Design review of the part built by this model. Coordinates are the model's own, in mm. Face numbers are marked on the shaded views. A direction names the side the tool comes from. Give positions to 0.01 mm unless a question says otherwise; leave off trailing zeros. Loops run counter-clockwise (first coordinate to the right, second up) from the corner with the lowest first, then second, coordinate; pieces in that order, holes last. Notation, with made-up numbers: (69, 37) -> (93, 37) arc R35 ccw to (93, 74) -> close; hole circle Ø11 at (-14.75, -34.5). An arc over 180 degrees is marked (long way). Use a Markdown table: item, result. Add a question column.
1. For pin 1 Ø4 at (x, y) = (-48.5, 7.5) entering from +Z; pin 2 Ø3.5 at (y, z) = (3, -6.5) entering from -X; pin 3 Ø3.5 at (x, y) = (46, -7.5) entering from +Z; pin 4 Ø3 at (x, y) = (5, 9.5) entering from -Z, all flat-tipped, find the tip position at first contact; note any pin that passes through.
2. Add section A-A (z = -4.5). State the section outline as (x, y) points.
3. Add section D-D (x = 48.5). State the section outline as (y, z) points.
4. Draft analysis for pull direction X (two halves, no side actions). For the marked faces 4, 5, 6 and 7, state which applies: pulls with the +X half, pulls with the -X half, needs draft (parallel to the pull), parting line crosses it, or undercut.
5. Add section C-C (z = -11.25). State the section outline as (x, y) points.
6. Add section B-B (x = 0). State the section outline as (y, z) points, and give its area (3 significant figures).
7. To check wall thickness, follow line 1 (Y direction, x = -48.5, z = -10.05); line 2 (X direction, y = 4, z = -4); line 3 (Y direction, x = 5.5, z = 2.8). State the ranges of each line that lie inside material, in increasing order.
8. For the marked faces 1, 2 and 3, list the 3-axis set-ups (+Z, -Z, +X, -X, +Y, -Y) from which the entire face can be reached by the end or side of a thin tool; tool diameter is ignored.
```python
from build123d import *

# Parameters (mm, degrees)
SKETCH1_W           = 85
SKETCH1_H           = 30
SKETCH1_R           = 6
BOSS_EXTRUDE1_DEPTH = 3.2
SKETCH5_R           = 1.75
CUT_EXTRUDE1_DEPTH  = 4.2
SKETCH7_R           = 3
CUT_EXTRUDE2_DEPTH  = 2
SKETCH2_W           = 4
SKETCH2_H           = 30
BOSS_EXTRUDE2_DEPTH = 12.3
SKETCH3_W           = 16
SKETCH3_H           = 30
SKETCH3_R           = 2.25
BOSS_EXTRUDE3_DEPTH = 4
CHAMFER1_SIZE       = 5


with BuildPart() as part:
    # Sketch1 → Boss-Extrude1 (new body)
    with BuildSketch(Plane.XY):
        Rectangle(SKETCH1_W, SKETCH1_H)
        Circle(SKETCH1_R, mode=Mode.SUBTRACT)
    extrude(amount=BOSS_EXTRUDE1_DEPTH)

    # Sketch5 → Cut-Extrude1 (cut, through all)
    with BuildSketch(Plane.XY.offset(3.2)):
        with Locations((5.5, 9.526279442)):
            Circle(SKETCH5_R)
        with Locations((-11, 0)):
            Circle(SKETCH5_R)
        with Locations((5.5, -9.526279442)):
            Circle(SKETCH5_R)
    extrude(amount=-CUT_EXTRUDE1_DEPTH, mode=Mode.SUBTRACT)

    # Sketch7 → Cut-Extrude2 (cut)
    with BuildSketch(Plane(origin=(0, 0, 0), x_dir=(-1, 0, 0), z_dir=(0, 0, -1))):
        with Locations((-5.5, 9.526279442)):
            Circle(SKETCH7_R)
        with Locations((11, 0)):
            Circle(SKETCH7_R)
        with Locations((-5.5, -9.526279442)):
            Circle(SKETCH7_R)
    extrude(amount=-CUT_EXTRUDE2_DEPTH, mode=Mode.SUBTRACT)

    # Sketch2 → Boss-Extrude2 (add)
    with BuildSketch(Plane(origin=(0, 0, 0), x_dir=(-1, 0, 0), z_dir=(0, 0, -1))):
        with Locations((40.5, 0)):
            Rectangle(SKETCH2_W, SKETCH2_H)
        with Locations((-40.5, 0)):
            Rectangle(SKETCH2_W, SKETCH2_H)
    extrude(amount=BOSS_EXTRUDE2_DEPTH)

    # Sketch3 → Boss-Extrude3 (add)
    with BuildSketch(Plane(origin=(0, 0, -12.3), x_dir=(-1, 0, 0), z_dir=(0, 0, -1))):
        with Locations((46.5, 0)):
            Rectangle(SKETCH3_W, SKETCH3_H)
        with Locations((48.5, -7.5)):
            Circle(SKETCH3_R, mode=Mode.SUBTRACT)
        with Locations((48.5, 7.5)):
            Circle(SKETCH3_R, mode=Mode.SUBTRACT)
        with Locations((-46.5, 0)):
            Rectangle(SKETCH3_W, SKETCH3_H)
        with Locations((-48.5, 7.5)):
            Circle(SKETCH3_R, mode=Mode.SUBTRACT)
        with Locations((-48.5, -7.5)):
            Circle(SKETCH3_R, mode=Mode.SUBTRACT)
    extrude(amount=-BOSS_EXTRUDE3_DEPTH)

    # Chamfer1
    chamfer1_edges = [part.edges().sort_by_distance(p)[0] for p in [
        (54.5, 15, -10.3),
        (54.5, -15, -10.3),
        (-54.5, -15, -10.3),
        (-54.5, 15, -10.3),
    ]]
    chamfer(chamfer1_edges, length=CHAMFER1_SIZE)


solid = part.part
```
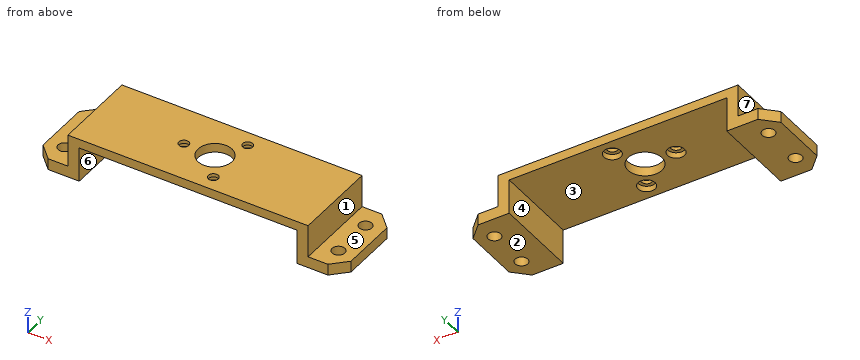
Taken from the geometry:
| question | item | result |
|---|---|---|
| 1 | pin 1 | passes through |
| 1 | pin 2 | stops at x = -42.5 |
| 1 | pin 3 | stops at z = -8.3 |
| 1 | pin 4 | stops at z = 2 |
| 2 | outline | (-42.5, -15) -> (-38.5, -15) -> (-38.5, 15) -> (-42.5, 15) -> close; (38.5, -15) -> (42.5, -15) -> (42.5, 15) -> (38.5, 15) -> close |
| 3 | outline | (-15, -12.3) -> (-9.75, -12.3) -> (-9.75, -8.3) -> (-15, -8.3) -> close; (-5.25, -12.3) -> (5.25, -12.3) -> (5.25, -8.3) -> (-5.25, -8.3) -> close; (9.75, -12.3) -> (15, -12.3) -> (15, -8.3) -> (9.75, -8.3) -> close |
| 4 | face 4 | undercut |
| 4 | face 5 | needs draft |
| 4 | face 6 | undercut |
| 4 | face 7 | pulls with the -X half |
| 5 | outline | (-54.5, -10) -> (-49.5, -15) -> (-38.5, -15) -> (-38.5, 15) -> (-49.5, 15) -> (-54.5, 10) -> close; (38.5, -15) -> (49.5, -15) -> (54.5, -10) -> (54.5, 10) -> (49.5, 15) -> (38.5, 15) -> close; hole circle Ø4.5 at (-48.5, -7.5); hole circle Ø4.5 at (-48.5, 7.5); hole circle Ø4.5 at (48.5, -7.5); hole circle Ø4.5 at (48.5, 7.5) |
| 6 | outline | (-15, 0) -> (-6, 0) -> (-6, 3.2) -> (-15, 3.2) -> close; (6, 0) -> (15, 0) -> (15, 3.2) -> (6, 3.2) -> close |
| 6 | area | 57.6 mm^2 |
| 7 | line 1 | y = -15 to -9.75, -5.25 to 5.25, 9.75 to 15 |
| 7 | line 2 | x = -42.5 to -38.5, 38.5 to 42.5 |
| 7 | line 3 | y = -15 to -11.28, -7.78 to -2.4, 2.4 to 7.78, 11.28 to 15 |
| 8 | face 1 | +Z, +X, +Y, -Y |
| 8 | face 2 | -Z, +X, -X, +Y, -Y |
| 8 | face 3 | -Z, +Y, -Y |
